Verification items for the finished model (mm, model axes). Round coordinates to 2 decimals unless told otherwise and drop trailing zeros. Write each loop counter-clockwise with the first axis right and the second up, starting at its lowest first coordinate (ties: lowest second). Pieces come first, ordered by that corner, then holes. Notation, with made-up numbers: M 71.5,24 L 94.5,24 A23 cw 94.5,61 Z; hole C 73.5,73.5 d10. An arc over 180 degrees is marked long. One line per question, with ' | ' between items.
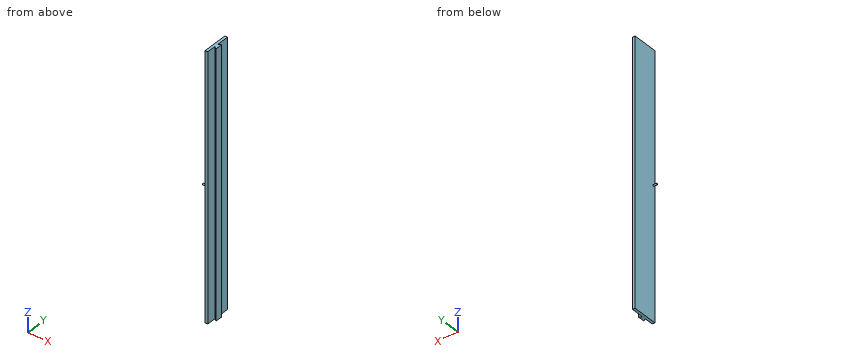
from build123d import *

# Parameters (mm, degrees)
BOSS_EXTRUDE1_DEPTH = 1500
SKETCH3_R           = 4
BOSS_EXTRUDE2_DEPTH = 20


with BuildPart() as part:
    # Sketch2 → Boss-Extrude1 (new body)
    with BuildSketch(Plane.XY):
        Polygon((0, -70), (0, -20), (15, -30), (15, 10), (0, 0), (0, 70), (-15, 70), (-15, -70), align=None)
    extrude(amount=BOSS_EXTRUDE1_DEPTH)

    # Sketch3 → Boss-Extrude2 (add)
    with BuildSketch(Plane.ZY.offset(15)):
        with Locations(Location((750, -60, 0), (0, 0, 90))):
            Circle(SKETCH3_R)
    extrude(amount=BOSS_EXTRUDE2_DEPTH)


solid = part.part
1. Section check A-A, the plane z = 635. Record the cut outline in (x, y).
Results:
outline: M -15,-70 L 0,-70 L 0,-20 L 15,-30 L 15,10 L 0,0 L 0,70 L -15,70 Z
2. Thickness scan on line 1 (X direction, y = 14.5, z = 446.5); line 2 (X direction, y = -24, z = 206); line 3 (X direction, y = -24.5, z = 1433). Record the ranges inside material, lowest first.
Results:
line 1: x = -15 to 0 | line 2: x = -15 to 0, 6 to 15 | line 3: x = -15 to 0, 6.75 to 15
3. Section check C-C, the plane x = -25. Record the cut outline in (y, z), then the cut area to 3 significant figures.
Results:
outline: C -60,750 d8 | area: 50.3 mm2
4. Section check B-B, the plane y = 27. Record the cut outline in (x, z).
Results:
outline: M -15,0 L 0,0 L 0,1500 L -15,1500 Z
5. Go/stop test with flat-tipped pins: P1, Ø6, axis at y = 47, z = 862, coming from the -X side; P2, Ø4, axis at x = 2.5, z = 234, coming from the -Y side; P3, Ø8, axis at x = -14.5, y = 40.5, coming from the -Z side. Record where each tip stops, or that it passes through.
Results:
P1: stops at x = -15 | P2: stops at y = -23 | P3: stops at z = 0
